The listing builds one solid part. Answer for the finished solid, in the listing's coordinates (mm). A direction names the side the tool comes from. Coordinates: 2 decimals unless noted, no trailing zeros. Write each loop counter-clockwise with the first axis right and the second up, starting at its lowest first coordinate (ties: lowest second). Pieces come first, ordered by that corner, then holes. Notation, with made-up numbers: M 26,33 L 69,33 A18 cw 69,56 Z; hole C -28.75,40 d2. An arc over 180 degrees is marked long. Answer as a JSON object with one key per item and string values. Group by question number.
from build123d import *

# Parameters (mm, degrees)
F0_R     = 32.1345484261
F1_DEPTH = 50.8
F2_R     = 30.48
F3_R     = 12.7
F4_DEPTH = 12.7
F5_R     = 5.08


with BuildPart() as f1:
    # F0 (on Front) → F1 (new body, symmetric)
    with BuildSketch(Plane.XZ):
        Circle(F0_R)
    extrude(amount=F1_DEPTH, both=True)

    # F2
    f2_edges = [f1.edges().sort_by_distance(p)[0] for p in [
        (-32.134548, -50.8, 0),
    ]]
    fillet(f2_edges, radius=F2_R)

    # F3
    f3_edges = [f1.edges().sort_by_distance(p)[0] for p in [
        (-32.134548, 50.8, 0),
    ]]
    fillet(f3_edges, radius=F3_R)

    # F4 (add): a face of the model
    f4_faces = [f1.faces().sort_by_distance(p)[0] for p in [
        (0, 50.8, 0),
    ]]
    extrude(f4_faces, amount=F4_DEPTH)

    # F5
    f5_edges = [f1.edges().sort_by_distance(p)[0] for p in [
        (-19.434548, 63.5, 0),
    ]]
    fillet(f5_edges, radius=F5_R)


solid = f1.part
Item 1: A cutting plane is placed at A-A, the plane y = -12.5. Write down the section's boundary in (x, z), and give its area (3 significant figures).
Item 2: Consider L1, parallel to X at y = 0, z = 27; L2, parallel to Y at x = 0, z = -3; L3, parallel to X at y = 8, z = -5. Determine where each line is inside the solid, lowest interval first. Write a range as from..to.
Item 3: A cutting plane is placed at B-B, the plane y = 42. Write down the section's boundary in (x, z), and give its area (3 significant figures).
Item 4: Flat-ended cylindrical pins translate along their axes: pin 1 Ø3 at (x, z) = (6, -24) entering from -Y; pin 2 Ø12 at (x, y) = (0.5, -35.5) entering from +Z; pin 3 Ø3 at (x, z) = (-6, -9) entering from -Y. Find the tip coordinate at first contact, or state that the pin passes through.
Item 5: A tool of negligible diameter and unlimited length cuts with its end or side. For faces 1 (the face through (-15.42, 54.56, -11.83)), 2 (the face through (-25.501, 8.481, -19.553)), from which of +Z, -Z, +X, -X, +Y, -Y can it reach the whole face along a straight path? Write none if from no direction.
Answer:
{
 "1": {"outline": "C 0,0 d64.27", "area": "3,240 mm2"},
 "2": {"L1": "-17.42..17.42", "L2": "-50.77..63.5", "L3": "-31.74..31.74"},
 "3": {"outline": "C 0,0 d63.04", "area": "3,120 mm2"},
 "4": {"pin 1": "y = -41.84", "pin 2": "z = 30.72", "pin 3": "y = -49.82"},
 "5": {"face 1": "+Y", "face 2": "+Y, -Y"}
}
